Design review of the part built by this model. Coordinates are the model's own, in mm. Round coordinates to 2 decimals unless told otherwise and drop trailing zeros. Write each loop counter-clockwise with the first axis right and the second up, starting at its lowest first coordinate (ties: lowest second). Pieces come first, ordered by that corner, then holes. Notation, with made-up numbers: M -9,5 L 12,5 A24 ccw 12,39 Z; hole C 76.5,32 d4. An arc over 180 degrees is marked long. One line per question, with ' | ' between items. Start each with the question number.
Item 1: Add section C-C, the plane z = 2.1. Give the number of separate pieces and of enclosed holes in the cut face, and give its area (3 significant figures).
Item 2: Add section A-A, the plane y = -13.5. State the section outline as (x, z) points.
Item 3: Add section B-B, the plane y = 61.5. State the section outline as (x, z) points, and give its area (3 significant figures).
Item 4: Add section D-D, the plane x = -90. State the section outline as (y, z) points, and give its area (3 significant figures).
Item 5: Insertion check: pin 1 Ø4 at (x, y) = (112.5, 67.9) entering from -Z; pin 2 Ø5 at (x, y) = (-80, -88) entering from +Z; pin 3 Ø1.5 at (x, z) = (94, 1) entering from +Y. Each pin has a flat end and moves straight along its axis. Give the tip position at first contact, or say it passes through.
Item 6: For L1, parallel to Y at x = -82.5, z = 1.55; L2, parallel to Y at x = -65, z = 1.6; L3, parallel to X at y = -88, z = 1.9, list the stretches that pass through material, from the lowest coordinate up.
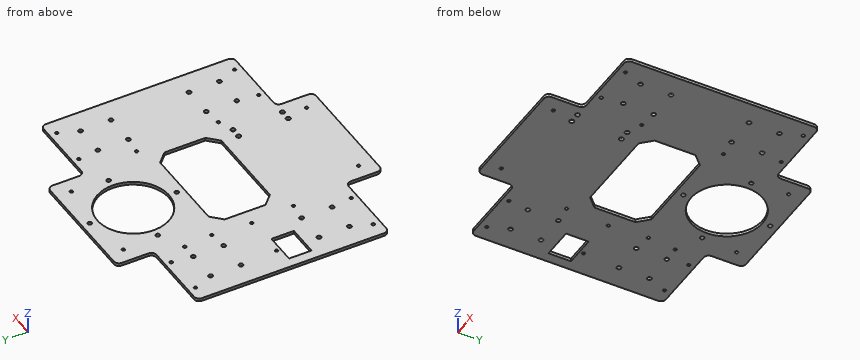
```python
from build123d import *

# Parameters (mm, degrees)
SKETCH_1_W          = 270
SKETCH_1_H          = 260
EXTRUDE_1_DEPTH     = 3
CUT_EXTRUDE_1_REACH = 189.441
SKETCH_2_W          = 75
SKETCH_2_H          = 36
FILLET_1_R          = 5
SKETCH_3_R          = 35
CUT_EXTRUDE_2_DEPTH = 10
SKETCH_4_R          = 2.1
CUT_EXTRUDE_3_DEPTH = 4.55
SKETCH_5_R          = 1.5
SKETCH_5_R_2        = 2.2
CUT_EXTRUDE_4_DEPTH = 188.440657276
SKETCH_6_R          = 1.5
CUT_EXTRUDE_5_DEPTH = 188.440657276
SKETCH_7_R          = 1.5
CUT_EXTRUDE_6_DEPTH = 188.440657276
SKETCH_8_W          = 104
SKETCH_8_H          = 60
CUT_EXTRUDE_7_DEPTH = 188.440657276
CHAMFER_1_SIZE      = 10
SKETCH_9_R          = 2
CUT_EXTRUDE_8_DEPTH = 188.440657276
CUT_EXTRUDE_9_REACH = 189.441
SKETCH_11_W         = 30.5
SKETCH_11_H         = 22


with BuildPart() as part:
    # 草图1 → 凸台-拉伸1 (new body)
    with BuildSketch(Plane.XY):
        Rectangle(SKETCH_1_W, SKETCH_1_H)
    extrude(amount=EXTRUDE_1_DEPTH)

    # 草图2 → 切除-拉伸1 (cut, up to next)
    with BuildSketch(Plane.XY.offset(3), mode=Mode.PRIVATE) as cut_extrude_1_sk1:
        with Locations((97.5, -112)):
            Rectangle(SKETCH_2_W, SKETCH_2_H)
    cut_extrude_1_tool1 = extrude(cut_extrude_1_sk1.sketch, amount=-CUT_EXTRUDE_1_REACH, mode=Mode.PRIVATE) & part.part
    # 草图2 → 切除-拉伸1 (cut, up to next)
    with BuildSketch(Plane.XY.offset(3), mode=Mode.PRIVATE) as cut_extrude_1_sk2:
        with Locations((-97.5, -112)):
            Rectangle(SKETCH_2_W, SKETCH_2_H)
    cut_extrude_1_tool2 = extrude(cut_extrude_1_sk2.sketch, amount=-CUT_EXTRUDE_1_REACH, mode=Mode.PRIVATE) & part.part
    # 草图2 → 切除-拉伸1 (cut, up to next)
    with BuildSketch(Plane.XY.offset(3), mode=Mode.PRIVATE) as cut_extrude_1_sk3:
        with Locations((-97.5, 112)):
            Rectangle(SKETCH_2_W, SKETCH_2_H)
    cut_extrude_1_tool3 = extrude(cut_extrude_1_sk3.sketch, amount=-CUT_EXTRUDE_1_REACH, mode=Mode.PRIVATE) & part.part
    # 草图2 → 切除-拉伸1 (cut, up to next)
    with BuildSketch(Plane.XY.offset(3), mode=Mode.PRIVATE) as cut_extrude_1_sk4:
        with Locations((97.5, 112)):
            Rectangle(SKETCH_2_W, SKETCH_2_H)
    cut_extrude_1_tool4 = extrude(cut_extrude_1_sk4.sketch, amount=-CUT_EXTRUDE_1_REACH, mode=Mode.PRIVATE) & part.part
    add(cut_extrude_1_tool1.solids().sort_by_distance((97.5, -112, 3))[0], mode=Mode.SUBTRACT)
    add(cut_extrude_1_tool2.solids().sort_by_distance((-97.5, -112, 3))[0], mode=Mode.SUBTRACT)
    add(cut_extrude_1_tool3.solids().sort_by_distance((-97.5, 112, 3))[0], mode=Mode.SUBTRACT)
    add(cut_extrude_1_tool4.solids().sort_by_distance((97.5, 112, 3))[0], mode=Mode.SUBTRACT)

    # 圆角1
    fillet_1_edges = [part.edges().sort_by_distance(p)[0] for p in [
        (60, 130, 1.5),
        (135, 94, 1.5),
        (60, 94, 1.5),
        (-135, 94, 1.5),
        (-60, 130, 1.5),
        (-60, 94, 1.5),
        (-60, -130, 1.5),
        (-135, -94, 1.5),
        (-60, -94, 1.5),
        (135, -94, 1.5),
        (60, -130, 1.5),
        (60, -94, 1.5),
    ]]
    fillet(fillet_1_edges, radius=FILLET_1_R)

    # 草图3 → 切除-拉伸2 (cut)
    with BuildSketch(Plane.XY.offset(3)):
        with Locations((0, 80)):
            Circle(SKETCH_3_R)
    extrude(amount=-CUT_EXTRUDE_2_DEPTH, mode=Mode.SUBTRACT)

    # 草图4 → 切除-拉伸3 (cut)
    with BuildSketch(Plane(origin=(0, 0, 0), x_dir=(-1, 0, 0), z_dir=(0, 0, -1))):
        with Locations((-112.5, -38.1)):
            Circle(SKETCH_4_R)
        with Locations((-112.5, -67.9)):
            Circle(SKETCH_4_R)
        with Locations((-82.5, -38.1)):
            Circle(SKETCH_4_R)
        with Locations((-82.5, -67.9)):
            Circle(SKETCH_4_R)
        with Locations((-82.5, 67.9)):
            Circle(SKETCH_4_R)
        with Locations((-82.5, 38.1)):
            Circle(SKETCH_4_R)
        with Locations((-112.5, 67.9)):
            Circle(SKETCH_4_R)
        with Locations((-112.5, 38.1)):
            Circle(SKETCH_4_R)
        with Locations((112.5, 38.1)):
            Circle(SKETCH_4_R)
        with Locations((112.5, 67.9)):
            Circle(SKETCH_4_R)
        with Locations((82.5, 38.1)):
            Circle(SKETCH_4_R)
        with Locations((82.5, 67.9)):
            Circle(SKETCH_4_R)
        with Locations((82.5, -67.9)):
            Circle(SKETCH_4_R)
        with Locations((82.5, -38.1)):
            Circle(SKETCH_4_R)
        with Locations((112.5, -67.9)):
            Circle(SKETCH_4_R)
        with Locations((112.5, -38.1)):
            Circle(SKETCH_4_R)
    extrude(amount=-CUT_EXTRUDE_3_DEPTH, mode=Mode.SUBTRACT)

    # 草图5 → 切除-拉伸4 (cut, through all)
    with BuildSketch(Plane(origin=(0, 0, 0), x_dir=(-1, 0, 0), z_dir=(0, 0, -1))):
        with Locations((45, 115)):
            Circle(SKETCH_5_R)
        with Locations((120, 87)):
            Circle(SKETCH_5_R)
        with Locations((120, -87)):
            Circle(SKETCH_5_R)
        with Locations((45, -115)):
            Circle(SKETCH_5_R)
        with Locations((65, -40)):
            Circle(SKETCH_5_R)
        with Locations((65, 40)):
            Circle(SKETCH_5_R)
        with Locations(Location((-65, 40, 0), (0, 0, 180))):
            Circle(SKETCH_5_R)
        with Locations(Location((-65, -40, 0), (0, 0, 180))):
            Circle(SKETCH_5_R)
        with Locations(Location((-45, -115, 0), (0, 0, 180))):
            Circle(SKETCH_5_R)
        with Locations(Location((-120, -87, 0), (0, 0, 180))):
            Circle(SKETCH_5_R)
        with Locations(Location((-120, 87, 0), (0, 0, 180))):
            Circle(SKETCH_5_R)
        with Locations(Location((-45, 115, 0), (0, 0, 180))):
            Circle(SKETCH_5_R)
        with Locations((-50, -94.25)):
            Circle(SKETCH_5_R_2)
        with Locations((-40, -94.25)):
            Circle(SKETCH_5_R_2)
        with Locations((-50, -45.75)):
            Circle(SKETCH_5_R_2)
        with Locations((-40, -45.75)):
            Circle(SKETCH_5_R_2)
    extrude(amount=-CUT_EXTRUDE_4_DEPTH, mode=Mode.SUBTRACT)

    # 草图6 → 切除-拉伸5 (cut, through all)
    with BuildSketch(Plane.XY.offset(3)):
        with Locations((-110.5, 2.25)):
            Circle(SKETCH_6_R)
        with Locations((-67.5, 2.25)):
            Circle(SKETCH_6_R)
        with Locations((-67.5, 67.75)):
            Circle(SKETCH_6_R)
    extrude(amount=-CUT_EXTRUDE_5_DEPTH, mode=Mode.SUBTRACT)

    # 草图7 → 切除-拉伸6 (cut, through all)
    with BuildSketch(Plane(origin=(0, 0, 0), x_dir=(-1, 0, 0), z_dir=(0, 0, -1))):
        with Locations((80, 88)):
            Circle(SKETCH_7_R)
        with Locations(Location((-80, 88, 0), (0, 0, 180))):
            Circle(SKETCH_7_R)
        with Locations(Location((80, -88, 0), (0, 0, 180))):
            Circle(SKETCH_7_R)
        with Locations((-80, -88)):
            Circle(SKETCH_7_R)
    extrude(amount=-CUT_EXTRUDE_6_DEPTH, mode=Mode.SUBTRACT)

    # 草图8 → 切除-拉伸7 (cut, through all)
    with BuildSketch(Plane(origin=(0, 0, 0), x_dir=(-1, 0, 0), z_dir=(0, 0, -1))):
        Rectangle(SKETCH_8_W, SKETCH_8_H)
    extrude(amount=-CUT_EXTRUDE_7_DEPTH, mode=Mode.SUBTRACT)

    # 倒角1
    chamfer_1_edges = [part.edges().sort_by_distance(p)[0] for p in [
        (52, -30, 1.5),
        (52, 30, 1.5),
        (-52, 30, 1.5),
        (-52, -30, 1.5),
    ]]
    chamfer(chamfer_1_edges, length=CHAMFER_1_SIZE)

    # 草图9 → 切除-拉伸8 (cut, through all)
    with BuildSketch(Plane.XY.offset(3)):
        with Locations((42.5, 80)):
            Circle(SKETCH_9_R)
        with Locations((0, 37.5)):
            Circle(SKETCH_9_R)
        with Locations((-42.5, 80)):
            Circle(SKETCH_9_R)
        with Locations((0, 122.5)):
            Circle(SKETCH_9_R)
    extrude(amount=-CUT_EXTRUDE_8_DEPTH, mode=Mode.SUBTRACT)

    # 草图11 → 切除-拉伸9 (cut, up to next)
    with BuildSketch(Plane(origin=(0, 0, 0), x_dir=(-1, 0, 0), z_dir=(0, 0, -1)), mode=Mode.PRIVATE) as cut_extrude_9_sk1:
        with Locations((109.75, -12.761545207)):
            Rectangle(SKETCH_11_W, SKETCH_11_H)
    cut_extrude_9_tool1 = extrude(cut_extrude_9_sk1.sketch, amount=-CUT_EXTRUDE_9_REACH, mode=Mode.PRIVATE) & part.part
    add(cut_extrude_9_tool1.solids().sort_by_distance((-109.75, -12.761545, 0))[0], mode=Mode.SUBTRACT)


solid = part.part
```
Computed values:
1) separate pieces: 1 | enclosed holes: 46 | area: 48,400 mm^2
2) outline: M -135,0 L -125,0 L -125,3 L -135,3 Z; M -94.5,0 L -52,0 L -52,3 L -94.5,3 Z; M 52,0 L 135,0 L 135,3 L 52,3 Z
3) outline: M -135,0 L -29.71,0 L -29.71,3 L -135,3 Z; M 29.71,0 L 135,0 L 135,3 L 29.71,3 Z | area: 632 mm^2
4) outline: M -94,0 L 94,0 L 94,3 L -94,3 Z | area: 564 mm^2
5) pin 1: passes through | pin 2: stops at z = 3 | pin 3: stops at y = 94
6) L1: y = -94 to -70, -65.8 to -40.2, -36 to 36, 40.2 to 65.8, 70 to 94 | L2: y = -94 to -41.5, -38.5 to 38.5, 41.5 to 94 | L3: x = -135 to -121.12, -118.88 to -81.5, -78.5 to 78.5, 81.5 to 118.88, 121.12 to 135
